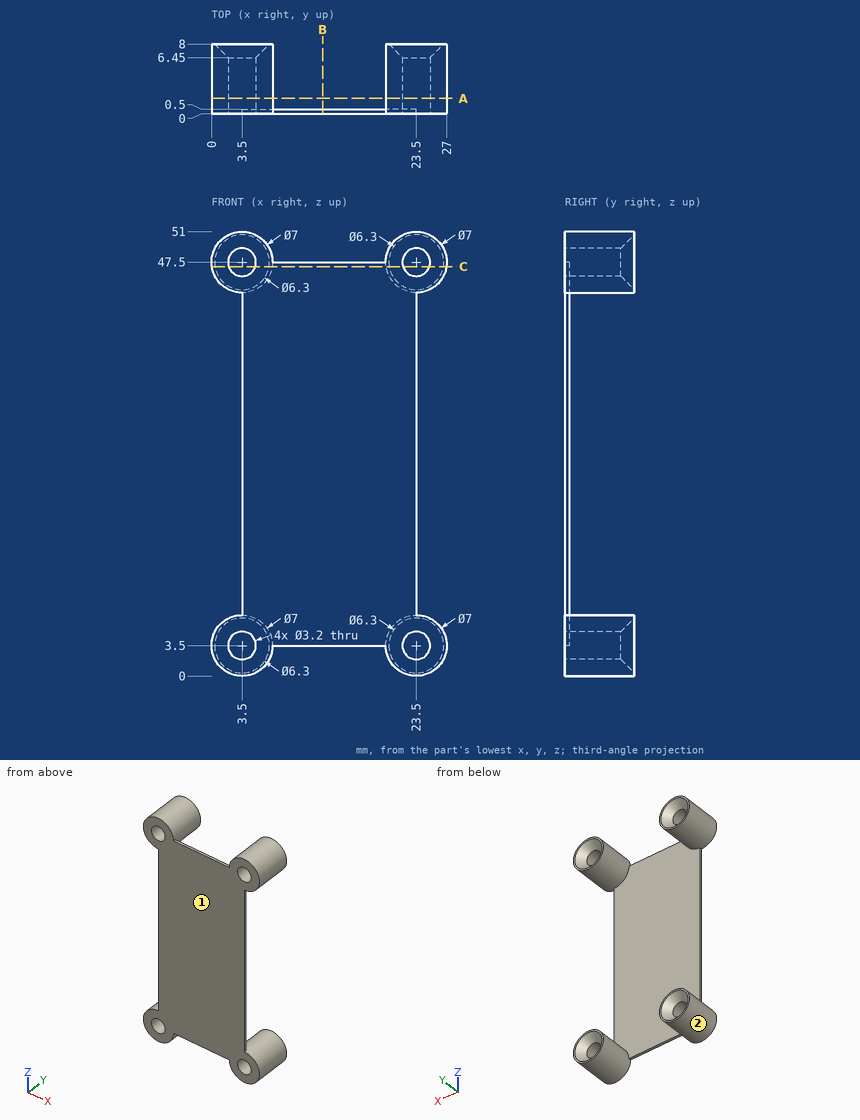
The figure shows three views and two pictorial views of one solid part (mm, origin at its lowest corner). Answer the questions. Give positions to 0.01 mm unless a question says otherwise; leave off trailing zeros. Write each loop counter-clockwise with the first axis right and the second up, starting at its lowest first coordinate (ties: lowest second). Pieces come first, ordered by that corner, then holes. Notation, with made-up numbers: M 37.5,-8 L 69.5,-8 A17 ccw 69.5,12 Z; hole C 24,-8 d7. An arc over 180 degrees is marked long. Write each question's results on one line, items separated by ' | '.
Q1. Section B-B, the plane x = 12.75 is taken. Write down the section's boundary in (y, z), then the cut area to 3 significant figures.
Output values:
outline: M 0,3.5 L 0.5,3.5 L 0.5,47.5 L 0,47.5 Z | area: 22.0 mm2
Q2. For a pull along X with two mould halves and no side action, classify the marked faces 1 and 2 as released by +X, released by -X, zero draft, split by the parting line, or undercut.
Output values:
face 1: zero draft | face 2: undercut
Q3. Section C-C, the plane z = 47 is taken. Count the separate pieces of the cut face and the enclosed holes in it, then the cut area to 3 significant figures.
Output values:
separate pieces: 3 | enclosed holes: 0 | area: 63.8 mm2
Q4. Section A-A, the plane y = 1.75 is taken. Write down the section's boundary in (x, z), then the cut area to 3 significant figures.
Output values:
outline: C 3.5,3.5 d7; C 3.5,47.5 d7; C 23.5,3.5 d7; C 23.5,47.5 d7; hole C 3.5,3.5 d3.2; hole C 3.5,47.5 d3.2; hole C 23.5,3.5 d3.2; hole C 23.5,47.5 d3.2 | area: 122 mm2
Q5. Consider L1, parallel to X at y = 4.5, z = 47.5; L2, parallel to Z at x = 23.5, y = 3; L3, parallel to Z at x = 4.5, y = 1.75. Determine where each line is inside the solid, lowest interval first. Write a range as from..to.
Output values:
L1: 0..1.9, 5.1..7, 20..21.9, 25.1..27 | L2: 0..1.9, 5.1..7, 44..45.9, 49.1..51 | L3: 0.15..2.25, 4.75..6.85, 44.15..46.25, 48.75..50.85
Q6. Flat-ended cylindrical pins translate along their axes: P1, Ø10, axis at x = 22, z = 29, coming from the +Y side; P2, Ø3.5, axis at x = 23.5, z = 47.5, coming from the +Y side; P3, Ø1, axis at x = 22.5, y = 1, coming from the +Z side. Find the tip coordinate at first contact, or state that the pin passes through.
Output values:
P1: y = 0.5 | P2: y = 6.6 | P3: z = 50.96
